Autodesk Inventor part; units mm, degrees
ref_plane "YZ Plane" through (0, 0, 0) normal (1, 0, 0) x (0, 1, 0)
ref_plane "XZ Plane" through (0, 0, 0) normal (0, 1, 0) x (-1, 0, 0)
ref_plane "XY Plane" through (0, 0, 0) normal (0, 0, 1) x (1, 0, 0)
sketch "Эскиз1" plane through (0, 0, 0) normal (0, 1, 0) x (-1, 0, 0)
  arc A0 (15, -25.7496) -> (-15, -25.7496) centre (0, 0) ccw
  line L0 (0, 0) -> (0, -429.8) construction
  line L1 (15, -25.7496) -> (15, -388.5878)
  line L2 (15, -388.5878) -> (0, -429.8)
  line L3 (0, 0) -> (0, -29.8) construction
  circle A1 centre (0, 0) radius 17.5 construction
  circle A2 centre (0, -17.5) radius 1.6 construction
  line L4 (12.3744, -12.3744) -> (0, 0) construction
  arc A3 (-4.9434, -18.4492) -> (13.5057, -13.5057) centre (0, 0) ccw
  arc A4 (-4.1152, -15.3582) -> (11.243, -11.243) centre (0, 0) ccw
  arc A5 (-4.1152, -15.3582) -> (-4.9434, -18.4492) centre (-4.5293, -16.9037) ccw
  line L5 (0, 0) -> (-4.5293, -16.9037) construction
  arc A6 (13.5057, -13.5057) -> (11.243, -11.243) centre (12.3744, -12.3744) ccw
  arc A7 (18.4492, -4.9434) -> (13.5057, 13.5057) centre (0, 0) ccw
  circle A8 centre (17.5, 0) radius 1.6 construction
  arc A9 (15.3582, -4.1152) -> (11.243, 11.243) centre (0, 0) ccw
  arc A10 (15.3582, -4.1152) -> (18.4492, -4.9434) centre (16.9037, -4.5293) ccw
  arc A11 (13.5057, 13.5057) -> (11.243, 11.243) centre (12.3744, 12.3744) ccw
  arc A12 (4.9434, 18.4492) -> (-13.5057, 13.5057) centre (0, 0) ccw
  circle A13 centre (0, 17.5) radius 1.6 construction
  arc A14 (4.1152, 15.3582) -> (-11.243, 11.243) centre (0, 0) ccw
  arc A15 (4.1152, 15.3582) -> (4.9434, 18.4492) centre (4.5293, 16.9037) ccw
  arc A16 (-13.5057, 13.5057) -> (-11.243, 11.243) centre (-12.3744, 12.3744) ccw
  arc A17 (-18.4492, 4.9434) -> (-13.5057, -13.5057) centre (0, 0) ccw
  circle A18 centre (-17.5, 0) radius 1.6 construction
  arc A19 (-15.3582, 4.1152) -> (-11.243, -11.243) centre (0, 0) ccw
  arc A20 (-15.3582, 4.1152) -> (-18.4492, 4.9434) centre (-16.9037, 4.5293) ccw
  arc A21 (-13.5057, -13.5057) -> (-11.243, -11.243) centre (-12.3744, -12.3744) ccw
  line L6 (-15, -25.7496) -> (-15, -388.5878)
  line L7 (-15, -388.5878) -> (0, -429.8)
  circle A22 centre (0, -229.8) radius 200
  line L8 (0, -29.8) -> (0, -229.8) construction
  circle A23 centre (0, -229.8) radius 210
  line L9 (0, -229.8) -> (71.8242, -32.4645) construction
  line L10 (71.8242, -32.4645) -> (63.991, -34.9344)
  line L11 (63.991, -34.9344) -> (68.404, -41.8615)
  line L12 (-71.8242, -32.4645) -> (-63.991, -34.9344)
  line L13 (-63.991, -34.9344) -> (-68.404, -41.8615)
  point P0 (-15, -30.3633)
  point P1 (15, -30.3633)
  point P2 (21.2626, -20.8792)
  point P3 (-21.2626, -20.8792)
  point P4 (-71.8242, -32.4645)
  point P5 (-68.404, -41.8615)
  dimension "d0" = 59.6
  dimension "d1" = 400
  dimension "d2" = 20
  dimension "d3" = 15
  dimension "d4" = 35
  dimension "d5" = 3.2
  dimension "d6" = 45
  dimension "d7" = 15
  dimension "d8" = 3.2
  dimension "d11" = 360
  dimension "d14" = 29.8
  dimension "d15" = 200
  dimension "d17" = 20
  dimension "d18" = 75
  dimension "d19" = 10
extrude "Выдавливание1" add sketch "Эскиз1" along normal blind 6 contours L1 A22 L6 A0 A23 | A0 A23 L10 L11 A22 L1 | A23 A0 | L1 L2 L7 L6 A22 | A0 L6 A22 L13 L12 A23
properties part number "клинок"
Source: CAD feature listing. Evaluate the final solid. Frame: model axes, mm. A direction names the side the tool comes from. Round coordinates to 2 decimals unless told otherwise and drop trailing zeros. Order: outer loops, then holes, each group sorted by start corner. A loop starts at its lowest first (then second) coordinate and runs counter-clockwise, first axis right, second up. Notation, with made-up numbers: (-21.5, 88.5) -> (21.5, 88.5) arc R27 cw to (21.5, 117.5) -> close; hole circle Ø1 at (36, 68.5). An arc over 180 degrees is marked (long way). One line per item, written item: value. Start each with the question number.
Q1. Draft query along Z for faces 3 (the flat face through (0, 0, -148)), 4 (the cylindrical face through (42.47, 2.96, -34.36)), 5 (the cylindrical face through (-46.548, 2.958, -25.024)). Return one class per face: pulls with the +Z half, pulls with the -Z half, needs draft (parallel to the pull), parting line crosses it, or undercut.
Q2. Section query D-D (x = 58). Return the cut outline in (y, z).
Q3. Section query A-A (z = 0). Return the cut outline in (x, y), plus the area to 3 significant figures.
Q4. Section query C-C (z = -163). Return the cut outline in (x, y), plus the area to 3 significant figures.
Q5. Material intervals for probe 1 along X at (y, z) = (4.55, -364); probe 2 along Z at (x, y) = (27.5, 1.9); probe 3 along Z at (x, y) = (-23, 2.5), sorted ascending.
Q6. Pin query (flat end, axial travel): pin 1 (1.8 mm diameter, centred on y = 4, z = -220.5, fed in from -X); pin 2 (3 mm diameter, centred on y = 1, z = -319.5, fed in from +X). Return the tip coordinate at first contact, or that it passes through.
Q7. Section query B-B (y = 1.35). Give the number of separate pieces and of enclosed holes in the cut face, plus the area to 3 significant figures.
Q8. Access query for faces 1 (the cylindrical face through (-41.72, 2.96, -34.2)), 2 (the flat face through (7.605, 2.958, -408.905)). Directions: +Z, -Z, +X, -X, +Y, -Y. A direction counts if a zero-diameter tool reaches every point of the face in a straight line with its end or side. Return the directions, or none.
Findings below:
1. face 3: needs draft
1. face 4: pulls with the -Z half
1. face 5: undercut
2. outline: (0, -38.39) -> (6, -38.39) -> (6, -27.97) -> (0, -27.97) -> close
3. outline: (-29.8, 0) -> (-19.1, 0) -> (-19.1, 6) -> (-29.8, 6) -> close; (-15.9, 0) -> (15.9, 0) -> (15.9, 6) -> (-15.9, 6) -> close; (19.1, 0) -> (29.8, 0) -> (29.8, 6) -> (19.1, 6) -> close
3. area: 319 mm²
4. outline: (-15, 0) -> (15, 0) -> (15, 6) -> (-15, 6) -> close
4. area: 180 mm²
5. probe 1: -15 to 15
5. probe 2: -31.7 to -21.61, -11.48 to 11.48
5. probe 3: -31.13 to -21.06, -18.95 to 18.95
6. pin 1: x = -15
6. pin 2: x = 15
7. separate pieces: 1
7. enclosed holes: 4
7. area: 15,000 mm²
8. face 1: -Z, +Y, -Y
8. face 2: -Z, +X, +Y, -Y
